```python
from build123d import *

# Parameters (mm, degrees)
BOSS_EXTRUDE1_DEPTH = 4.7625
SKETCH2_R           = 13.97
BOSS_EXTRUDE2_DEPTH = 4.7625
SKETCH3_R           = 3
CUT_EXTRUDE1_DEPTH  = 1.5875
CUT_EXTRUDE4_START  = 9.525
CUT_EXTRUDE4_DEPTH  = 3
CUT_EXTRUDE2_REACH  = 44.963
SKETCH4_R           = 1.6
SKETCH5_R           = 1.375
CUT_EXTRUDE3_DEPTH  = 12.7
CIRPATTERN3_COUNT   = 3
FILLET1_R           = 3
SKETCH7_R           = 4.7625
F_3_8IN_ROUND_DEPTH = 30.826926541


with BuildPart() as part:
    # Sketch1 → Boss-Extrude1 (new body)
    with BuildSketch(Plane(origin=(0, 0, 0), x_dir=(0, 0, -1), z_dir=(1, 0, 0))):
        Polygon((-10.815213918, 18.7325), (-21.630427835, 0), (-10.815213918, -18.7325), (10.815213918, -18.7325), (21.630427835, 0), (10.815213918, 18.7325), align=None)
    extrude(amount=BOSS_EXTRUDE1_DEPTH)

    # Sketch2 → Boss-Extrude2 (add)
    with BuildSketch(Plane(origin=(4.7625, 0, 0), x_dir=(0, 0, -1), z_dir=(1, 0, 0))):
        with Locations(Location((0, 0, 0), (0, 0, 180))):
            Circle(SKETCH2_R)
    extrude(amount=BOSS_EXTRUDE2_DEPTH)

    # Sketch3 → Cut-Extrude1 (cut)
    with BuildSketch(Plane.XZ.offset(18.7325)):
        with Locations((4.7625, 0)):
            Circle(SKETCH3_R)
    cut_extrude1 = extrude(amount=-CUT_EXTRUDE1_DEPTH, mode=Mode.SUBTRACT)

    # Sketch6 → Cut-Extrude4 (cut)
    with BuildSketch(Plane(origin=(0, 0, 0), x_dir=(-1, 0, 0), z_dir=(0, -1, 0)).offset(CUT_EXTRUDE4_START)):
        Polygon((-6.35021324, 2.75), (-9.525, 2.75), (-9.525, -2.75), (-6.35021324, -2.75), (-3.17478676, -2.75), (-1.587073519, 0), (-3.17478676, 2.75), align=None)
    cut_extrude4 = extrude(amount=CUT_EXTRUDE4_DEPTH, mode=Mode.SUBTRACT)

    # Cut-Extrude2: up to this face of the body (flat: up to its plane)
    cut_extrude2_end = Plane(part.part.faces().sort_by_distance((5.938262705, -9.525, 0))[0])
    # Sketch4 → Cut-Extrude2 (cut, up to the picked face)
    with BuildSketch(Plane.XZ.offset(17.145), mode=Mode.PRIVATE) as cut_extrude2_sk1:
        with Locations(Location((4.7625, 0, 0), (0, 0, 270))):
            Circle(SKETCH4_R)
    cut_extrude2_tool1 = split(extrude(cut_extrude2_sk1.sketch, amount=-CUT_EXTRUDE2_REACH, mode=Mode.PRIVATE), bisect_by=cut_extrude2_end, keep=Keep.BOTH, mode=Mode.PRIVATE)
    cut_extrude2 = cut_extrude2_tool1.solids().sort_by(Axis((4.7625, -17.145, 0), (0, 1, 0)))[0]
    add(cut_extrude2, mode=Mode.SUBTRACT)

    # Sketch5 → Cut-Extrude3 (cut)
    with BuildSketch(Plane.XZ.offset(17.145)):
        with Locations(Location((4.7625, 0, 0), (0, 0, 270))):
            Circle(SKETCH5_R)
    cut_extrude3 = extrude(amount=-CUT_EXTRUDE3_DEPTH, mode=Mode.SUBTRACT)

    # CirPattern3: Cut-Extrude1, Cut-Extrude4, Cut-Extrude2, Cut-Extrude3 ×3 about axis
    cirpattern3_axis = Axis((0, 0, 0), (1, 0, 0))
    add([cut_extrude1.rotate(cirpattern3_axis, i * 360 / CIRPATTERN3_COUNT) for i in range(1, CIRPATTERN3_COUNT)], mode=Mode.SUBTRACT)
    add([cut_extrude4.rotate(cirpattern3_axis, i * 360 / CIRPATTERN3_COUNT) for i in range(1, CIRPATTERN3_COUNT)], mode=Mode.SUBTRACT)
    add([cut_extrude2.rotate(cirpattern3_axis, i * 360 / CIRPATTERN3_COUNT) for i in range(1, CIRPATTERN3_COUNT)], mode=Mode.SUBTRACT)
    add([cut_extrude3.rotate(cirpattern3_axis, i * 360 / CIRPATTERN3_COUNT) for i in range(1, CIRPATTERN3_COUNT)], mode=Mode.SUBTRACT)

    # Fillet1
    fillet1_edges = [part.edges().sort_by_distance(p)[0] for p in [
        (2.38125, 18.7325, -10.815213918),
        (2.38125, 0, -21.630427835),
        (2.38125, -18.7325, -10.815213918),
        (2.38125, -18.7325, 10.815213918),
        (2.38125, 0, 21.630427835),
        (2.38125, 18.7325, 10.815213918),
    ]]
    fillet(fillet1_edges, radius=FILLET1_R)

    # Sketch7 → 3/8in Round (cut, through all)
    with BuildSketch(Plane(origin=(9.525, 0, 0), x_dir=(0, 0, -1), z_dir=(1, 0, 0))):
        Circle(SKETCH7_R)
    extrude(amount=-F_3_8IN_ROUND_DEPTH, mode=Mode.SUBTRACT)


solid = part.part
```
Geometry check sheet. Reference: the model listing, model coordinates, mm. A direction names the side the tool comes from. Coordinates: 2 decimals unless noted, no trailing zeros. Loops run counter-clockwise (first coordinate to the right, second up) from the corner with the lowest first, then second, coordinate; pieces in that order, holes last. Notation, with made-up numbers: (16, 21) - (30, 21) arc R18 cw to (30, 26) - close; hole circle Ø10 at (21, -5). An arc over 180 degrees is marked (long way). One line per item, written item: value. Start each with the question number.
(1) Material ranges on line 1 (X direction, y = -7.05, z = 0) (1 decimal); line 2 (Z direction, x = 3.25, y = 5); line 3 (Y direction, x = 8.5, z = 1) (3 decimals), recorded low to high. Write a range as [from, to].
(2) Tool access check on faces 1 (the flat face through (6, -11, 2.75)), 2 (the cylindrical face through (1.763, -17.95, 0.066)), 3 (the cylindrical face through (2.415, -0.022, -21.166)). Record the directions out of +Z, -Z, +X, -X, +Y, -Y that give a thin tool (end or side, any length) a straight path to the whole face; none if there is none.
(3) Mould release check, pull along X, two halves, no side actions. Record for faces 4 (the cylindrical face through (3.42, 3.28, -6.28)), 5 (the flat face through (1.29, 9.256, -16.286)), 6 (the cylindrical face through (1.763, 8.918, -15.578)): released by +X, released by -X, zero draft, split by the parting line, or undercut.
(4) Cross-section at A-A on y = 0. Enter the section's corners in (x, z) (1 decimal).
(5) Depth check by flat-ended pin: P1, Ø1.6, axis at x = 6, z = -1, coming from the +Y side; P2, Ø5, axis at y = 15.5, z = 6.5, coming from the +X side; P3, Ø1.5, axis at x = 3.5, y = -2, coming from the -Z side. Enter the tip coordinate at first touch or a pass-through.
(6) Cross-section at B-B on x = 8.75. Count the separate pieces of the cut face and the enclosed holes in it, plus the area to 3 significant figures.
Results below:
1. line 1: x = [0, 3.4], [6.1, 9.5]
1. line 2: z = [-18.74, -11.58], [-8.11, 8.11], [11.58, 18.74]
1. line 3: y = [-13.934, -12.525], [-9.525, -4.656], [4.656, 13.934]
2. face 1: +X
2. face 2: +X, -Y
2. face 3: -Z, +X, -X
3. face 4: undercut
3. face 5: zero draft
3. face 6: released by +X
4. outline: (0, -21.2) - (4.8, -21.2) - (4.8, -14) - (9.5, -14) - (9.5, -4.8) - (0, -4.8) - close; (0, 4.8) - (9.5, 4.8) - (9.5, 14) - (4.8, 14) - (4.8, 21.2) - (0, 21.2) - close
5. P1: stops at y = 13.97
5. P2: stops at x = 4.76
5. P3: stops at z = -20.89
6. separate pieces: 1
6. enclosed holes: 4
6. area: 492 mm2
